from build123d import *

# Parameters (mm, degrees)
SKETCH_1_R          = 50
EXTRUDE_1_DEPTH     = 8
FILLET_1_R          = 15
HOLE_WIZARD_M12_1_D = 10.2
FILLET_2_R          = 5


with BuildPart() as part:
    # 草图1 → 凸台-拉伸1 (new body)
    with BuildSketch(Plane.XY):
        with BuildLine():
            Line((0, 75), (310, 75))
            Line((310, 75), (310, 14.478023217))
            Line((310, 14.478023217), (632.18201609, -54.043305358))
            ThreePointArc((632.18201609, -54.043305358), (667.638820417, -94.015546308), (716.293570548, -71.932061317))
            Line((716.293570548, -71.932061317), (948, -121.211138337))
            Line((948, -121.211138337), (1008, -163))
            Line((1008, -163), (1008, -168))
            Line((1008, -168), (998.615528128, -168))
            ThreePointArc((998.615528128, -168), (933.656897839, -200.339106398), (984, -252.598206242))
            Line((984, -252.598206242), (978, -260))
            Line((978, -260), (861.968512478, -260))
            Line((861.968512478, -260), (-15.601965972, -73.359243847))
            ThreePointArc((-15.601965972, -73.359243847), (-74.588683084, 7.844001258), (0, 75))
        make_face()
        Circle(SKETCH_1_R, mode=Mode.SUBTRACT)
    extrude(amount=EXTRUDE_1_DEPTH)

    # 圆角1
    fillet_1_edges = [part.edges().sort_by_distance(p)[0] for p in [
        (310, 75, 4),
        (310, 14.478023217, 4),
    ]]
    fillet(fillet_1_edges, radius=FILLET_1_R)

    # M12 螺纹孔1 (through all)
    with Locations(Plane.XY.offset(8)):
        with Locations((75, 0)):
            Hole(HOLE_WIZARD_M12_1_D / 2)

    # 圆角2
    fillet_2_edges = [part.edges().sort_by_distance(p)[0] for p in [
        (632.18201609, -54.043305358, 4),
        (716.293570548, -71.932061317, 4),
    ]]
    fillet(fillet_2_edges, radius=FILLET_2_R)


solid = part.part
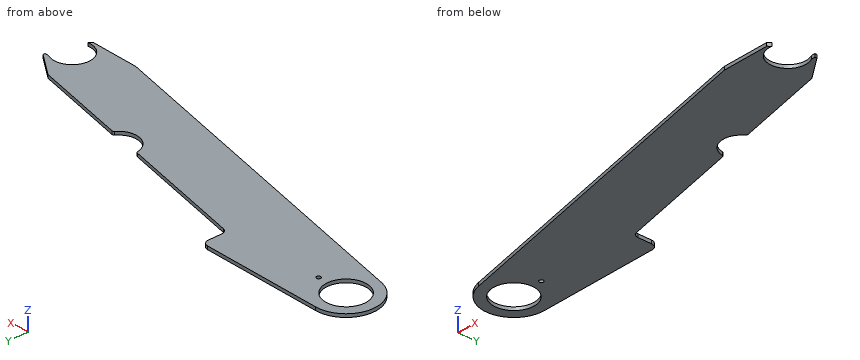
Build history of the part. All positions in model axes, mm. Coordinates: 2 decimals unless noted, no trailing zeros. Order: outer loops, then holes, each group sorted by start corner. A loop starts at its lowest first (then second) coordinate and runs counter-clockwise, first axis right, second up. Notation, with made-up numbers: (41.25, 27) - (51.25, 27) arc R18 ccw to (51.25, 53) - close; hole circle Ø4 at (72.5, 1). An arc over 180 degrees is marked (long way). Write each question's results on one line, items separated by ' | '. Start each with the question number.
Item 1: Flat gauge pins, fed straight in: pin 1 (1.5 mm diameter, centred on x = 503.5, z = 4.5, fed in from +Y); pin 2 (4 mm diameter, centred on y = 45.5, z = 4.5, fed in from +X); pin 3 (4 mm diameter, centred on y = -14, z = 2, fed in from -X). Where does each tip first touch, or does it go through?
Item 2: Band-saw the part on D-D on x = 222. Write the cut outline in (y, z).
Item 3: Band-saw the part on B-B on x = 14. Write the cut outline in (y, z).
Item 4: Band-saw the part on A-A on z = 1.5. Write the cut outline in (x, y).
Item 5: Band-saw the part on C-C on y = -208. Write the cut outline in (x, z).
Item 6: Wall check: probe 1 along X at (y, z) = (25, 5.5); probe 2 along Y at (x, z) = (0, 5); probe 3 along Y at (x, z) = (978, 2.5). Give the ranges that are in metal, low to high. Write a range as [from, to].
Numbers:
1) pin 1: y = -26.52 | pin 2: x = 310 | pin 3: x = -74.03
2) outline: (-123.89, 0) - (75, 0) - (75, 8) - (-123.89, 8) - close
3) outline: (-79.65, 0) - (-48, 0) - (-48, 8) - (-79.65, 8) - close; (48, 0) - (75, 0) - (75, 8) - (48, 8) - close
4) outline: (-15.6, -73.36) - (861.97, -260) - (978, -260) - (984, -252.6) arc R45 cw (long way) to (998.62, -168) - (1008, -168) - (1008, -163) - (948, -121.21) - (719.76, -72.67) arc R5 ccw to (714.55, -74.8) arc R45 cw to (632.61, -57.38) arc R5 ccw to (628.72, -53.31) - (321.88, 11.95) arc R15 cw to (310, 26.62) - (310, 60) arc R15 ccw to (295, 75) - (0, 75) arc R75 ccw to start; hole circle Ø100 at (0, 0); hole circle Ø10.2 at (75, 0)
5) outline: (617.47, 0) - (933, 0) - (933, 8) - (617.47, 8) - close
6) probe 1: [-70.71, -43.3], [43.3, 310.09] | probe 2: [-76.68, -50], [50, 75] | probe 3: [-260, -253], [-163, -142.11]
